```python
from build123d import *

# Parameters (mm, degrees)
F0_W     = 81
F0_H     = 162
F1_DEPTH = 12
F3_DEPTH = 160
F5_DEPTH = 7.431314


with BuildPart() as f1:
    # F0 (on Top) → F1 (new body)
    with BuildSketch(Plane.XY):
        with Locations((-32.540516, 31.026223)):
            Rectangle(F0_W, F0_H)
    extrude(amount=F1_DEPTH)

    # F2 (on face) → F3 (cut)
    with BuildSketch(Plane.XZ.offset(49.973777)):
        Polygon((6.709484, 7.660007), (6.709484, 10.115228), (-71.790516, 10.115228), (-71.790516, 7.937757), (-71.790516, 2.615228), (6.709484, 2.615228), align=None)
    extrude(amount=-F3_DEPTH, mode=Mode.SUBTRACT)

    # F4 (on face) → F5 (cut)
    with BuildSketch(Plane.XY.offset(12)):
        Polygon((5.959484, 108.026223), (-71.040516, 108.026223), (-71.040516, -44.254787), (-71.040516, -49.973777), (5.959484, -49.973777), (5.959484, -43.884151), align=None)
    extrude(amount=-F5_DEPTH, mode=Mode.SUBTRACT)


solid = f1.part
```
Design review of the part built by this model. Coordinates are the model's own, in mm. A direction names the side the tool comes from. Give positions to 0.01 mm unless a question says otherwise; leave off trailing zeros. Loops run counter-clockwise (first coordinate to the right, second up) from the corner with the lowest first, then second, coordinate; pieces in that order, holes last. Notation, with made-up numbers: M -9,72.25 L 31,72.25 A31 cw 31,105.25 Z; hole C 60.25,23.5 d3. An arc over 180 degrees is marked long. Return JSON: item names as keys, results as strings. Group by question number.
Item 1: Insertion check: pin 1 Ø2 at (x, z) = (-32, 11.5) entering from -Y; pin 2 Ø8 at (x, y) = (-34, 1.5) entering from +Z; pin 3 Ø3 at (x, z) = (-13.5, 3.5) entering from -Y. Each pin has a flat end and moves straight along its axis. Give the tip position at first contact, or say it passes through.
Item 2: Mouldability with a two-part tool opening along Z and no side actions: class faces 3 (the flat face through (7.959, 30, 6)), 4 (the flat face through (-33, 32, 0)), 5 (the flat face through (-33, 110.026, 6)) as released by +Z, released by -Z, zero draft, split by the parting line, or undercut.
Item 3: For probe 1 along X at (y, z) = (-5, 8); probe 2 along X at (y, z) = (12.5, 11.25); probe 3 along Z at (x, y) = (-44, 67), list the stretches that pass through material, from the lowest coordinate up.
Item 4: We need section C-C (y = -8.5). Give the boundary of the cut face in (x, z).
Item 5: Tool access review of faces 1 (the flat face through (6.709, 29, 6)), 2 (the flat face through (-33, -49.974, 2)): name each direction out of +Z, -Z, +X, -X, +Y, -Y from which nothing blocks a thin tool from reaching the whole face with its end or side.
Item 6: We need section B-B (x = -63). Give the boundary of the cut face in (y, z).
Item 7: We need section A-A (z = 5.75). Give the boundary of the cut face in (x, y).
Output:
{
 "1": {"pin 1": "stops at y = 108.03", "pin 2": "stops at z = 2.62", "pin 3": "stops at y = -49.97"},
 "2": {"face 3": "zero draft", "face 4": "released by -Z", "face 5": "undercut"},
 "3": {"probe 1": "x = -73.04 to -71.79, 6.71 to 7.96", "probe 2": "x = -73.04 to -71.04, 5.96 to 7.96", "probe 3": "z = 0 to 2.62"},
 "4": {"outline": "M -73.04,0 L 7.96,0 L 7.96,12 L 5.96,12 L 5.96,10.12 L 6.71,10.12 L 6.71,2.62 L -71.79,2.62 L -71.79,10.12 L -71.04,10.12 L -71.04,12 L -73.04,12 Z"},
 "5": {"face 1": "-Y", "face 2": "+Z, -Z, +X, -X, -Y"},
 "6": {"outline": "M -49.97,0 L 112.03,0 L 112.03,12 L 108.03,12 L 108.03,10.12 L 110.03,10.12 L 110.03,2.62 L -49.97,2.62 Z"},
 "7": {"outline": "M -73.04,-49.97 L -71.79,-49.97 L -71.79,110.03 L 6.71,110.03 L 6.71,-49.97 L 7.96,-49.97 L 7.96,112.03 L -73.04,112.03 Z"}
}
